Input: part model. Units: mm. Frame: model coordinates. Face numbers are marked on the shaded views. A direction names the side the tool comes from. Coordinates: 2 decimals unless noted, no trailing zeros. Write each loop counter-clockwise with the first axis right and the second up, starting at its lowest first coordinate (ties: lowest second). Pieces come first, ordered by that corner, then holes.
1) Draft query along Y for the marked faces 1, 2, 3 and 4. Return one class per face: pulls with the +Y half, pulls with the -Y half, needs draft (parallel to the pull), parting line crosses it, or undercut.
2) Section query D-D (z = -3.75). Output: boundary loops of the cut face in (x, y).
3) Pin query (flat end, axial travel): pin 1 Ø1.6 at (x, y) = (0, 0) entering from -Z. Return the tip coordinate at first contact, or that it passes through.
4) Set-up query: the marked faces 5 and 6. Return all of +Z, -Z, +X, -X, +Y, -Y with unobstructed straight access to the full face (end or side cutting, diameter ignored); none if empty.
5) Section query C-C (y = -0.5). Output: boundary loops of the cut face in (x, z).
6) Section query B-B (x = -2.5). Output: boundary loops of the cut face in (y, z), then the cut area to 3 significant figures.
7) Section query A-A (z = 8.25). Output: boundary loops of the cut face in (x, y), then the cut area to 3 significant figures.
8) Line query: L1, parallel to X at y = -0.75, z = -11.5; L2, parallel to Y at x = -1.5, z = 10.5; L3, parallel to Y at x = 2, z = 5.5. Output: solid intervals per line, ascending.
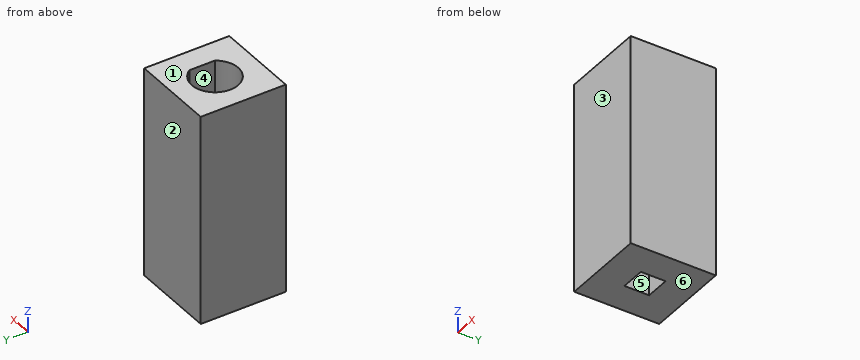
from build123d import *

# Parameters (mm, degrees)
F0_W     = 11
F0_H     = 11
F1_DEPTH = 14.2
F2_W     = 11
F2_H     = 11
F3_DEPTH = 3
F4_W     = 11
F4_H     = 11
F4_W_2   = 3.2
F4_H_2   = 3.2
F5_DEPTH = 10


# Not quite as in the source:
# - a feature names something its author has since deleted; it is built from what else it names


with BuildPart() as f1:
    # F0 (on Top) → F1 (new body)
    with BuildSketch(Plane.XY):
        Rectangle(F0_W, F0_H)
        with BuildLine():
            ThreePointArc((2.5, 1.6583123952), (2.8722813233, 0.8660254038), (3, 0))
            ThreePointArc((3, 0), (2.8722813233, -0.8660254038), (2.5, -1.6583123952))
            ThreePointArc((2.5, -1.6583123952), (-0.8660254038, -2.8722813233), (-3, 0))
            ThreePointArc((-3, 0), (-0.8660254038, 2.8722813233), (2.5, 1.6583123952))
        make_face(mode=Mode.SUBTRACT)
        with BuildLine():
            ThreePointArc((2.5, -1.6583123952), (2.8722813233, -0.8660254038), (3, 0))
            ThreePointArc((3, 0), (2.8722813233, 0.8660254038), (2.5, 1.6583123952))
            Line((2.5, 1.6583123952), (2.5, 0))
            Line((2.5, 0), (2.5, -1.6583123952))
        make_face()
    extrude(amount=F1_DEPTH)

    # F2 (on face) → F3 (join)
    with BuildSketch(Plane(origin=(0, 0, 0), x_dir=(1, 0, 0), z_dir=(0, 0, -1))):
        Rectangle(F2_W, F2_H)
        with BuildLine():
            ThreePointArc((2.5, -1.6583123952), (-3, 0), (2.5, 1.6583123952))
            Line((2.5, 1.6583123952), (2.5, -1.6583123952))
        make_face(mode=Mode.SUBTRACT)
        with BuildLine():
            Line((2.5, -1.6583123952), (2.5, 1.6583123952))
            ThreePointArc((2.5, 1.6583123952), (-3, 0), (2.5, -1.6583123952))
        make_face()
    extrude(amount=F3_DEPTH)

    # F4 (on face) → F5 (join)
    with BuildSketch(Plane(origin=(0, 0, -3), x_dir=(1, 0, 0), z_dir=(0, 0, -1))):
        Rectangle(F4_W, F4_H)
        Rectangle(F4_W_2, F4_H_2, mode=Mode.SUBTRACT)
    extrude(amount=F5_DEPTH)


solid = f1.part
Answer:
1. face 1: needs draft
1. face 2: pulls with the +Y half
1. face 3: pulls with the -Y half
1. face 4: undercut
2. outline: (-5.5, -5.5) - (5.5, -5.5) - (5.5, 5.5) - (-5.5, 5.5) - close; hole (-1.6, -1.6) - (1.6, -1.6) - (1.6, 1.6) - (-1.6, 1.6) - close
3. pin 1: stops at z = -3
4. face 5: -Z
4. face 6: -Z, +X, -X, +Y, -Y
5. outline: (-5.5, -13) - (-1.6, -13) - (-1.6, -3) - (1.6, -3) - (1.6, -13) - (5.5, -13) - (5.5, 14.2) - (2.5, 14.2) - (2.5, 0) - (-2.96, 0) - (-2.96, 14.2) - (-5.5, 14.2) - close
6. outline: (-5.5, -13) - (5.5, -13) - (5.5, 14.2) - (1.66, 14.2) - (1.66, 0) - (-1.66, 0) - (-1.66, 14.2) - (-5.5, 14.2) - close
6. area: 252 mm2
7. outline: (-5.5, -5.5) - (5.5, -5.5) - (5.5, 5.5) - (-5.5, 5.5) - close; hole (2.5, -1.66) - (2.5, 1.66) arc R3 ccw (long way) to start
7. area: 93.9 mm2
8. L1: x = -5.5 to -1.6, 1.6 to 5.5
8. L2: y = -5.5 to -2.6, 2.6 to 5.5
8. L3: y = -5.5 to -2.24, 2.24 to 5.5
